The listing builds one solid part. Answer for the finished solid, in the listing's coordinates (mm). A direction names the side the tool comes from. Coordinates: 2 decimals unless noted, no trailing zeros. Write each loop counter-clockwise with the first axis right and the second up, starting at its lowest first coordinate (ties: lowest second). Pieces come first, ordered by that corner, then holes.
(1) The part is cut by section A-A on x = -25. Determine the outline of the cut face in (y, z).
(2) The part is cut by section C-C on y = 15. Determine the outline of the cut face in (x, z), plus the area to 3 significant figures.
(3) The part is cut by section D-D on z = 18. Determine the outline of the cut face in (x, y).
(4) The part is cut by section B-B on y = 4.5. Determine the outline of the cut face in (x, z).
(5) Which of the six approach directions +Z, -Z, +X, -X, +Y, -Y give full straight-line access (tool end or side, diameter ignored) to faces 5 (the flat face through (0, -13, 12)), 6 (the flat face through (0, 15, 25))?
(6) For a pull along X with two mould halves and no side action, classify faces 1 (the flat face through (0, -22, 12)), 2 (the flat face through (32, 0, 12)), 3 (the cylindrical face through (16.14, 12.1, 12.68)), 4 (the cylindrical face through (-31.14, 21.1, 12.68)) as +X half, -X half, draft (parallel to the pull), parting line (faces both ways), or undercut.
(7) Given P1, Ø3, axis at x = 25, y = 16.07, coming from the +Z side; P2, Ø6, axis at x = 23.5, y = 16.5, coming from the -Z side, each flat-ended and moving along its own axis, determine where each tip first touches the part or whether it passes through.
(8) Straight lines are drawn through the part: line 1 (Y direction, x = 25, z = 15); line 2 (X direction, y = -9.5, z = 8.5); line 3 (Y direction, x = 3, z = 5.75). For each, find the intervals that lie inside material, in ascending order.
from build123d import *

# Parameters (mm, degrees)
SKETCH_1_W      = 64
SKETCH_1_H      = 44
SKETCH_1_R      = 2.5
SKETCH_1_W_2    = 34
SKETCH_1_H_2    = 26
EXTRUDE_1_DEPTH = 25
FILLET_1_R      = 3


with BuildPart() as part:
    # 草图1 → 凸台-拉伸1 (new body)
    with BuildSketch(Plane.XY):
        Rectangle(SKETCH_1_W, SKETCH_1_H)
        with Locations((-25, 16.06779661)):
            Circle(SKETCH_1_R, mode=Mode.SUBTRACT)
        with Locations((-25, -15.93220339)):
            Circle(SKETCH_1_R, mode=Mode.SUBTRACT)
        with Locations((25, -15.93220339)):
            Circle(SKETCH_1_R, mode=Mode.SUBTRACT)
        with Locations((25, 16.06779661)):
            Circle(SKETCH_1_R, mode=Mode.SUBTRACT)
        Rectangle(SKETCH_1_W_2, SKETCH_1_H_2, mode=Mode.SUBTRACT)
    extrude(amount=EXTRUDE_1_DEPTH)

    # 圆角1
    fillet_1_edges = [part.edges().sort_by_distance(p)[0] for p in [
        (17, -13, 12.5),
        (17, 13, 12.5),
        (-17, 13, 12.5),
        (-17, -13, 12.5),
        (32, -22, 12.5),
        (-32, -22, 12.5),
        (-32, 22, 12.5),
        (32, 22, 12.5),
    ]]
    fillet(fillet_1_edges, radius=FILLET_1_R)


solid = part.part
Model answer:
1. outline: (-22, 0) - (-18.43, 0) - (-18.43, 25) - (-22, 25) - close; (-13.43, 0) - (13.57, 0) - (13.57, 25) - (-13.43, 25) - close; (18.57, 0) - (22, 0) - (22, 25) - (18.57, 25) - close
2. outline: (-32, 0) - (-27.26, 0) - (-27.26, 25) - (-32, 25) - close; (-22.74, 0) - (22.74, 0) - (22.74, 25) - (-22.74, 25) - close; (27.26, 0) - (32, 0) - (32, 25) - (27.26, 25) - close
2. area: 1,370 mm2
3. outline: (-32, -19) arc R3 ccw to (-29, -22) - (29, -22) arc R3 ccw to (32, -19) - (32, 19) arc R3 ccw to (29, 22) - (-29, 22) arc R3 ccw to (-32, 19) - close; hole circle Ø5 at (-25, -15.93); hole circle Ø5 at (-25, 16.07); hole (-17, -10) arc R3 ccw to (-14, -13) - (14, -13) arc R3 ccw to (17, -10) - (17, 10) arc R3 ccw to (14, 13) - (-14, 13) arc R3 ccw to (-17, 10) - close; hole circle Ø5 at (25, -15.93); hole circle Ø5 at (25, 16.07)
4. outline: (-32, 0) - (-17, 0) - (-17, 25) - (-32, 25) - close; (17, 0) - (32, 0) - (32, 25) - (17, 25) - close
5. face 5: +Z, -Z
5. face 6: +Z, +X, -X, +Y, -Y
6. face 1: draft
6. face 2: +X half
6. face 3: undercut
6. face 4: -X half
7. P1: passes through
7. P2: stops at z = 0
8. line 1: y = -22 to -18.43, -13.43 to 13.57, 18.57 to 22
8. line 2: x = -32 to -17, 17 to 32
8. line 3: y = -22 to -13, 13 to 22
